Geometry check sheet. Reference: the model listing, model coordinates, mm. A direction names the side the tool comes from. Round coordinates to 2 decimals unless told otherwise and drop trailing zeros. Loops run counter-clockwise (first coordinate to the right, second up) from the corner with the lowest first, then second, coordinate; pieces in that order, holes last. Notation, with made-up numbers: (73.5, 77) -> (90.5, 77) arc R9 ccw to (90.5, 87) -> close; hole circle Ø8 at (-25, 42). An arc over 180 degrees is marked (long way). Use a Markdown table: item, result. Add a question column.
Q1. Sectioned sample at A-A, the plane z = 0.5. Enter the section's corners in (x, y) (3 decimals), then the cut area to 3 significant figures.
Q2. Release check for a two-part mould opening along Z. For faces 1 (the face through (2, -4, -2.75)), 2 (the face through (2, -4, -2.25)), 3 (the face through (-8.34, 0.62, 0.06)) record: released by +Z, released by -Z, zero draft, split by the parting line, or undercut.
Q3. Sectioned sample at B-B, the plane y = 2.25. Enter the section's corners in (x, z) (3 decimals), then the cut area to 3 significant figures.
Q4. Sectioned sample at D-D, the plane z = -1.5. Enter the section's corners in (x, y) (3 decimals).
Q5. Gauge pin test, flat ends, axial feed: P1, Ø1.2, axis at y = 2.5, z = 0, coming from the -X side (3 decimals); P2, Ø0.6, axis at y = -4, z = 2.5, coming from the +X side (3 decimals); P3, Ø0.6, axis at y = -4, z = -2.5, coming from the -X side (3 decimals). Record the tip position at first contact, or that the pin passes through.
Q6. Material ranges on L1, parallel to X at y = 2.25, z = -1.5 (3 decimals); L2, parallel to X at y = 2.5, z = -3 (3 decimals); L3, parallel to Y at x = -5.75, z = 0.25, recorded low to high.
Q7. Set-up check for faces 4 (the face through (-8.624, -3.693, 0.033)), 5 (the face through (6.567, -1.947, 2.539)), 6 (the face through (3.525, 0, -3.4)): record each of +Z, -Z, +X, -X, +Y, -Y from which the full face is reachable in a straight line by a thin tool's end or side.
Q8. Sectioned sample at C-C, the plane x = 1.5. Enter the section's corners in (y, z).
```python
from build123d import *

# Parameters (mm, degrees)
SKETCH1_W               = 19.05
SKETCH1_H               = 6.4
BOSS_EXTRUDE1_DEPTH     = 3.95
SKETCH2_OUTSIDE_W       = 14.218
SKETCH2_OUTSIDE_H       = 12.718
SKETCH2_OUTSIDE_R       = 3.2
CUT_EXTRUDE1_DEPTH      = 6
SKETCH3_R               = 0.75
SKETCH3_W               = 1.2
SKETCH3_H               = 0.5
BOSS_EXTRUDE2_DEPTH     = 1
CUT_EXTRUDE2_DEPTH      = 1
CUT_EXTRUDE2_DEPTH_BACK = 8.9


with BuildPart() as part:
    # Sketch1 → Boss-Extrude1 (new body, symmetric)
    with BuildSketch(Plane.XY):
        Rectangle(SKETCH1_W, SKETCH1_H)
    extrude(amount=BOSS_EXTRUDE1_DEPTH, both=True)

    # Sketch2 outside → Cut-Extrude1 (cut)
    with BuildSketch(Plane(origin=(9.525, 0, 0), x_dir=(0, 0, -1), z_dir=(1, 0, 0))):
        Rectangle(SKETCH2_OUTSIDE_W, SKETCH2_OUTSIDE_H)
        Circle(SKETCH2_OUTSIDE_R, mode=Mode.SUBTRACT)
    extrude(amount=-CUT_EXTRUDE1_DEPTH, mode=Mode.SUBTRACT)

    # Sketch3 → Boss-Extrude2 (add)
    with BuildSketch(Plane.XZ.offset(3.2)):
        with Locations((-7.875, 0)):
            Circle(SKETCH3_R)
        with Locations((2.325, 2.5)):
            Rectangle(SKETCH3_W, SKETCH3_H)
        with Locations((2.325, -2.5)):
            Rectangle(SKETCH3_W, SKETCH3_H)
    extrude(amount=BOSS_EXTRUDE2_DEPTH)

    # Sketch5 → Cut-Extrude2 (cut, two sides)
    with BuildSketch(Plane.XY.offset(3.95)) as cut_extrude2_sk:
        with BuildLine():
            Line((-5.575, 53.392661022), (-5.575, 3.2))
            Line((-5.575, 3.2), (-5.575, 1.75))
            ThreePointArc((-5.575, 1.75), (-8.368071786, 0.593071786), (-9.525, -2.2))
            Line((-9.525, -2.2), (-9.525, -3.2))
            Line((-9.525, -3.2), (-9.525, -53.392661022))
            Line((-9.525, -53.392661022), (-109.841715444, -49.681935442))
            Line((-109.841715444, -49.681935442), (-105.891715444, 57.103386601))
            Line((-105.891715444, 57.103386601), (-5.575, 53.392661022))
        make_face()
    extrude(amount=CUT_EXTRUDE2_DEPTH, mode=Mode.SUBTRACT)
    extrude(cut_extrude2_sk.sketch, amount=-CUT_EXTRUDE2_DEPTH_BACK, mode=Mode.SUBTRACT)


solid = part.part
```
Values:
| question | item | result |
|---|---|---|
| 1 | outline | (-9.525, -3.2) -> (-8.434, -3.2) -> (-8.434, -4.2) -> (-7.316, -4.2) -> (-7.316, -3.2) -> (3.525, -3.2) -> (3.525, -3.161) -> (9.525, -3.161) -> (9.525, 3.161) -> (3.525, 3.161) -> (3.525, 3.2) -> (-5.575, 3.2) -> (-5.575, 1.75) arc R3.95 ccw to (-9.525, -2.2) -> close |
| 1 | area | 113 mm^2 |
| 2 | face 1 | released by -Z |
| 2 | face 2 | undercut |
| 2 | face 3 | zero draft |
| 3 | outline | (-5.575, -3.95) -> (3.525, -3.95) -> (3.525, -2.275) -> (9.525, -2.275) -> (9.525, 2.275) -> (3.525, 2.275) -> (3.525, 3.95) -> (-5.575, 3.95) -> close |
| 3 | area | 99.2 mm^2 |
| 4 | outline | (-9.525, -3.2) -> (3.525, -3.2) -> (3.525, -2.827) -> (9.525, -2.827) -> (9.525, 2.827) -> (3.525, 2.827) -> (3.525, 3.2) -> (-5.575, 3.2) -> (-5.575, 1.75) arc R3.95 ccw to (-9.525, -2.2) -> close |
| 5 | P1 | x = -5.575 |
| 5 | P2 | x = 2.925 |
| 5 | P3 | x = 1.725 |
| 6 | L1 | -5.575 to 9.525 |
| 6 | L2 | -5.575 to 3.525 |
| 6 | L3 | -3.2 to 1.75 |
| 7 | face 4 | -Y |
| 7 | face 5 | +X |
| 7 | face 6 | -Z, +X |
| 8 | outline | (-3.2, -3.95) -> (3.2, -3.95) -> (3.2, 3.95) -> (-3.2, 3.95) -> close |
